```python
from build123d import *

# Parameters (mm, degrees)
DODANIE_WYCI_GNI_CIE1_DEPTH = 2
OTW_R1_D                    = 6
OTW_R1_DEPTH                = 2


with BuildPart() as part:
    # Szkic1 → Dodanie-wyciągnięcie1 (new body)
    with BuildSketch(Plane(origin=(0, 0, 0), x_dir=(1, 0, 0), z_dir=(0, 1, 0))):
        with BuildLine():
            Line((-6, 0), (-6, -15))
            Line((-6, -15), (6, -15))
            Line((6, -15), (6, 0))
            ThreePointArc((6, 0), (0, 6), (-6, 0))
        make_face()
    extrude(amount=DODANIE_WYCI_GNI_CIE1_DEPTH)

    # Otwór1
    with Locations(Plane(origin=(0, 2, 0), x_dir=(1, 0, 0), z_dir=(0, 1, 0))):
        with Locations((0, 0)):
            Hole(OTW_R1_D / 2, depth=OTW_R1_DEPTH)


solid = part.part
```
Geometry: final body of the model. Coordinates: model frame, mm. Give positions to 0.01 mm unless a question says otherwise; leave off trailing zeros. Write each loop counter-clockwise with the first axis right and the second up, starting at its lowest first coordinate (ties: lowest second). Pieces come first, ordered by that corner, then holes.
1. Line query: probe 1 along Z at (x, y) = (0, 1.25); probe 2 along Z at (x, y) = (2, 0.6); probe 3 along Z at (x, y) = (-5.5, 0.25). Output: solid intervals per line, ascending.
2. Section query C-C, the plane z = 2.25. Return loops of the section in (x, y).
3. Draft query along Z for faces 1 (the flat face through (6, 1, 8)), 2 (the cylindrical face through (3, 1, 0)), 3 (the flat face through (0, 1, 15)). Return one class per face: released by +Z, released by -Z, zero draft, split by the parting line, or undercut.
4. Section query A-A, the plane x = 0. Return loops of the section in (y, z).
5. Section query B-B, the plane y = 0.85. Return loops of the section in (x, z).
Computed:
1. probe 1: z = -6 to -3, 3 to 15
1. probe 2: z = -5.66 to -2.24, 2.24 to 15
1. probe 3: z = -2.4 to 15
2. outline: (-6, 0) - (-1.98, 0) - (-1.98, 2) - (-6, 2) - close; (1.98, 0) - (6, 0) - (6, 2) - (1.98, 2) - close
3. face 1: zero draft
3. face 2: undercut
3. face 3: released by +Z
4. outline: (0, -6) - (2, -6) - (2, -3) - (0, -3) - close; (0, 3) - (2, 3) - (2, 15) - (0, 15) - close
5. outline: (-6, 0) arc R6 ccw to (6, 0) - (6, 15) - (-6, 15) - close; hole circle Ø6 at (0, 0)
